Can you work these out from the model? Positions are in its coordinate system, mm. A direction names the side the tool comes from. Give positions to 0.01 mm unless a question says otherwise; leave off trailing zeros. Write each loop counter-clockwise with the first axis right and the second up, starting at its lowest first coordinate (ties: lowest second). Pieces come first, ordered by that corner, then holes.
1. Suppose I cut it at C-C (y = 23.5). Please give me the cut outline in (x, z), and give its area (3 significant figures).
2. Suppose I cut it at A-A (y = 51). Please give me the cut outline in (x, z), and give its area (3 significant figures).
3. On a 3-axis mill with a long thin cutter (end or side, diameter ignored), from which of +Z, -Z, +X, -X, +Y, -Y can I reach the whole of each face in a straight line? I mean faces 1 (the flat face through (24, 49.5, -2)), 2 (the flat face through (26.25, 51, -4.4)), 3 (the cylindrical face through (-23.67, 2.03, 3.11)). Say none if no direction works.
4. Suppose I cut it at B-B (y = 29.5). Please give me the cut outline in (x, z), and give its area (3 significant figures).
5. I'm going to push flat-ended pins straight in: pin 1 (1.5 mm diameter, centred on y = 46.5, z = 2, fed in from -X); pin 2 (1.5 mm diameter, centred on x = 22.5, y = 51, fed in from -Z); pin 3 (6 mm diameter, centred on y = 48.5, z = -10, fed in from -X). Where does each tip first touch, or does it pass through?
6. If I drill on probe 1 along Y at (x, z) = (-22.5, -3); probe 2 along Y at (x, z) = (3.5, 22.5); probe 3 along Y at (x, z) = (25, -3), over which ranges is the centre line in solid material (lowest first)?
7. Thinking about a two-plate mould opening in Z: for faces 4 (the cylindrical face through (11.49, 38.739, -27.712)), 5 (the cylindrical face through (-0.385, 31.731, -17.496)), 6 (the flat face through (-26.25, 51, -1)), which applies, pulls with the +Z half, pulls with the -Z half, needs draft (parallel to the pull), parting line crosses it, or undercut?
```python
from build123d import *

# Parameters (mm, degrees)
CUT_EXTRUDE3_DEPTH           = 25
CUT_EXTRUDE3_DEPTH_BACK      = 40
CUT_EXTRUDE5_DEPTH           = 2
CUT_EXTRUDE5_DEPTH_BACK      = 5
BOSS_EXTRUDE2_DEPTH          = 5
CUT_EXTRUDE6_DEPTH           = 22
SKETCH17_W                   = 7
SKETCH17_H                   = 20.303986046
CUT_REVOLVE1_ANGLE           = 45
CUT_REVOLVE1_OTHER_WAY_ANGLE = 45
SKETCH14_R                   = 1
CUT_EXTRUDE7_DEPTH           = 10
CUT_EXTRUDE8_START           = -10
SKETCH15_R                   = 1
CUT_EXTRUDE8_DEPTH           = 10


with BuildPart() as part:
    # Sketch1 → Revolve1 (revolve)
    with BuildSketch(Plane.XY, mode=Mode.PRIVATE) as revolve1_sk:
        with BuildLine():
            Line((20.9, 0), (23.871591838, 0))
            Line((23.871591838, 0), (23.871591838, 4))
            Line((23.871591838, 4), (22.9, 4.236662843))
            Line((22.9, 4.236662843), (22.9, 11.874576818))
            ThreePointArc((22.9, 11.874576818), (23.83692213, 16.100759435), (26.472123903, 19.535021249))
            Line((26.472123903, 19.535021249), (26.427876097, 19.497892931))
            ThreePointArc((26.427876097, 19.497892931), (29.06307787, 22.932154745), (30, 27.158337362))
            Line((30, 27.158337362), (30, 50))
            ThreePointArc((30, 50), (28.828427125, 52.828427125), (26, 54))
            Line((26, 54), (0, 54))
            Line((0, 54), (0, 15))
            Line((0, 15), (19.9, 15))
            ThreePointArc((19.9, 15), (20.607106781, 14.707106781), (20.9, 14))
            Line((20.9, 14), (20.9, 0))
        make_face()
    revolve(revolve1_sk.sketch.rotate(Axis((0, 0, 0), (0, 1, 0)), 90), axis=Axis((0, 0, 0), (0, 1, 0)))

    # Sketch11 → Cut-Extrude3 (cut, two sides: drawn at the far end of the back side and taken through both)
    with BuildSketch(Plane(origin=(0, 19.535021249, 0), x_dir=(-1, 0, 0), z_dir=(0, -1, 0)).offset(-CUT_EXTRUDE3_DEPTH_BACK)):
        with BuildLine():
            Line((-17.5, 0), (17.5, 0))
            ThreePointArc((17.5, 0), (0, 17.5), (-17.5, 0))
        make_face()
    extrude(amount=CUT_EXTRUDE3_DEPTH + CUT_EXTRUDE3_DEPTH_BACK, mode=Mode.SUBTRACT)

    # Sketch9 → Cut-Extrude5 (cut, two sides: drawn at the far end of the back side and taken through both)
    with BuildSketch(Plane(origin=(0, 50, 0), x_dir=(-1, 0, 0), z_dir=(0, -1, 0)).offset(-CUT_EXTRUDE5_DEPTH_BACK)):
        with BuildLine():
            Line((-30, 0), (30, 0))
            ThreePointArc((30, 0), (0, 30), (-30, 0))
        make_face()
    extrude(amount=CUT_EXTRUDE5_DEPTH + CUT_EXTRUDE5_DEPTH_BACK, mode=Mode.SUBTRACT)

    # Sketch13 → Boss-Extrude2 (add)
    with BuildSketch(Plane(origin=(0, 0, 0), x_dir=(-1, 0, 0), z_dir=(0, 0, -1))):
        with BuildLine():
            Line((21.75, 52.5), (25.75, 52.5))
            ThreePointArc((25.75, 52.5), (26.103553391, 52.353553391), (26.25, 52))
            Line((26.25, 52), (26.25, 50))
            ThreePointArc((26.25, 50), (26.103553391, 49.646446609), (25.75, 49.5))
            Line((25.75, 49.5), (21.75, 49.5))
            ThreePointArc((21.75, 49.5), (21.396446609, 49.646446609), (21.25, 50))
            Line((21.25, 50), (21.25, 52))
            ThreePointArc((21.25, 52), (21.396446609, 52.353553391), (21.75, 52.5))
        make_face()
        with BuildLine():
            Line((-25.75, 52.5), (-21.75, 52.5))
            ThreePointArc((-21.75, 52.5), (-21.396446609, 52.353553391), (-21.25, 52))
            Line((-21.25, 52), (-21.25, 50))
            ThreePointArc((-21.25, 50), (-21.396446609, 49.646446609), (-21.75, 49.5))
            Line((-21.75, 49.5), (-25.75, 49.5))
            ThreePointArc((-25.75, 49.5), (-26.103553391, 49.646446609), (-26.25, 50))
            Line((-26.25, 50), (-26.25, 52))
            ThreePointArc((-26.25, 52), (-26.103553391, 52.353553391), (-25.75, 52.5))
        make_face()
    extrude(amount=BOSS_EXTRUDE2_DEPTH)

    # Sketch16 → Cut-Extrude6 (cut)
    with BuildSketch(Plane(origin=(0, 50, 0), x_dir=(-1, 0, 0), z_dir=(0, -1, 0))):
        with BuildLine():
            Line((27.95979256, -1.5), (-27.95979256, -1.5))
            ThreePointArc((-27.95979256, -1.5), (0, -28), (27.95979256, -1.5))
        make_face()
    extrude(amount=CUT_EXTRUDE6_DEPTH, mode=Mode.SUBTRACT)

    # Sketch17 → Cut-Revolve1 (revolve, cut)
    with BuildSketch(Plane(origin=(0, 0, 0), x_dir=(0, 0, -1), z_dir=(1, 0, 0))):
        with Locations((-28.883918314, 38.580330385)):
            Rectangle(SKETCH17_W, SKETCH17_H)
    revolve(axis=Axis((0, 0, 0), (0, 0.9999633813881498, 0.008557796607647805)), revolution_arc=CUT_REVOLVE1_ANGLE, mode=Mode.SUBTRACT)

    # Sketch17 → Cut-Revolve1 other way (revolve, cut)
    with BuildSketch(Plane(origin=(0, 0, 0), x_dir=(0, 0, -1), z_dir=(1, 0, 0))):
        with Locations((-28.883918314, 38.580330385)):
            Rectangle(SKETCH17_W, SKETCH17_H)
    revolve(axis=Axis((0, 0, 0), (0, -0.9999633813881498, -0.008557796607647805)), revolution_arc=CUT_REVOLVE1_OTHER_WAY_ANGLE, mode=Mode.SUBTRACT)

    # Sketch14 → Cut-Extrude7 (cut)
    with BuildSketch(Plane.ZY.offset(-21.25)):
        with Locations(Location((-3, 51, 0), (0, 0, 270))):
            Circle(SKETCH14_R)
    extrude(amount=-CUT_EXTRUDE7_DEPTH, mode=Mode.SUBTRACT)

    # Sketch15 → Cut-Extrude8 (cut)
    with BuildSketch(Plane(origin=(-21.25, 0, 0), x_dir=(0, 0, -1), z_dir=(1, 0, 0)).offset(CUT_EXTRUDE8_START)):
        with Locations(Location((3, 51, 0), (0, 0, 270))):
            Circle(SKETCH15_R)
    extrude(amount=CUT_EXTRUDE8_DEPTH, mode=Mode.SUBTRACT)


solid = part.part
```
Checks:
1. outline: circle Ø58.61 at (0, 0); hole (-17.5, 0) arc R17.5 ccw to (17.5, 0) - close
1. area: 2,220 mm2
2. outline: (-29.87, 0) - (-26.25, 0) - (-26.25, -2) - (-21.25, -2) - (-21.25, 0) - (21.25, 0) - (21.25, -2) - (26.25, -2) - (26.25, 0) - (29.87, 0) arc R29.87 ccw to start; (-26.25, -5) - (-21.25, -5) - (-21.25, -4) - (-26.25, -4) - close; (21.25, -5) - (26.25, -5) - (26.25, -4) - (21.25, -4) - close
2. area: 1,430 mm2
3. face 1: -Z, +X, -X
3. face 2: -Z, +X, +Y
3. face 3: -Y
4. outline: (-27.96, 1.5) arc R28 cw to (-19.67, 19.93) - (-21.09, 21.34) arc R30 ccw (long way) to (21.09, 21.34) - (19.67, 19.93) arc R28 cw to (27.96, 1.5) - close; hole (-17.5, 0) arc R17.5 ccw to (17.5, 0) - close
4. area: 1,110 mm2
5. pin 1: stops at x = -29.97
5. pin 2: stops at z = -5
5. pin 3: stops at x = -29.16
6. probe 1: y = 0 to 48, 49.5 to 50, 52 to 52.5
6. probe 2: y = 0 to 28, 50 to 54
6. probe 3: y = 18.23 to 48, 49.5 to 50, 52 to 52.5
7. face 4: parting line crosses it
7. face 5: undercut
7. face 6: needs draft
